```python
from build123d import *

# Parameters (mm, degrees)
F1_DEPTH = 63.4248778224
F2_R     = 5.3887909161
F3_DEPTH = 102.1241396666
F6_DEPTH = 25


with BuildPart() as f1:
    # F0 (on Top) → F1 (new body)
    with BuildSketch(Plane.XY):
        Polygon((-32.9633839428, -48.3821220696), (34.9777191877, -14.2513811588), (49.3006780744, 44.1745221615), (0, 63.3342713118), align=None)
    extrude(amount=F1_DEPTH)

    # F2 (on face) → F3 (cut)
    with BuildSketch(Plane(origin=(12.7649742408, -25.4101261271, 0), x_dir=(0.8935828585, 0.4488982902, 0), z_dir=(0.4488982902, -0.8935828585, 0))):
        with Locations((17.1215422451, 26.0495916009)):
            Circle(F2_R)
    extrude(amount=-F3_DEPTH, mode=Mode.SUBTRACT)

    # F5 (on face) → F6 (cut)
    with BuildSketch(Plane(origin=(36.2904519106, -8.8965103003, 0), x_dir=(0.2380972915, 0.9712413087, 0), z_dir=(0.9712413087, -0.2380972915, 0))):
        Polygon((48.6116707325, 8.5855266079), (41.9424623251, 42.4769595265), (-16.6801717132, 35.93596071), align=None)
    extrude(amount=-F6_DEPTH, mode=Mode.SUBTRACT)


solid = f1.part
```
Model file for the job. Use its own axes, mm. A direction names the side the tool comes from. Coordinates: 2 decimals unless noted, no trailing zeros. Order: outer loops, then holes, each group sorted by start corner. A loop starts at its lowest first (then second) coordinate and runs counter-clockwise, first axis right, second up. Notation, with made-up numbers: (80.5, 52.5) - (108.5, 52.5) arc R23 ccw to (108.5, 83.5) - close; hole circle Ø9 at (15.5, 38). An arc over 180 degrees is marked (long way). Return JSON: item names as keys, results as strings. Group by question number.
1) Flat gauge pins, fed straight in: P1, Ø3, axis at x = 6, z = 28, coming from the +Y side; P2, Ø2, axis at x = -11.5, z = 55, coming from the -Y side; P3, Ø5, axis at y = -7, z = 34.5, coming from the -X side. Where does each tip first touch, or does it go through?
2) Probe line 1 (X direction, y = 27.5, z = 21.5); line 2 (X direction, y = 8, z = 16.5); line 3 (X direction, y = 4, z = 14). List the from-to ranges inside material, lowest first. Write a range as from..to.
3) Mould opens along X. For faces 1 (the flat face through (8, 8, 0)), 2 (the flat face through (0.532, -31.556, 31.268)), 3 (the cylindrical face through (9.6, 16.42, 20.79)) say: released by +X, released by -X, zero draft, split by the parting line, or undercut.
4) Tool access for faces 4 (the flat face through (42.04, 14.55, 45.36)), 5 (the flat face through (35.11, 38.06, 25.29)): list every direction of +Z, -Z, +X, -X, +Y, -Y with a clear straight run to the whole face (end or side of a thin tool).
5) Saw through at C-C, the plane y = -38.5. Write the cut outline in (x, z).
6) Saw through at D-D, the plane z = 51. Write the cut outline in (x, y), plus the area to 3 significant figures.
7) Saw through at B-B, the plane z = 38.5. Write the cut outline in (x, y), plus the area to 3 significant figures.
8) Saw through at A-A, the plane x = 43.5. Write the cut outline in (y, z).
Values found:
{
 "1": {"P1": "stops at y = 61.59", "P2": "stops at y = -38.1", "P3": "stops at x = -21.49"},
 "2": {"line 1": "x = -10.57..2.11, 8.58..19.47", "line 2": "x = -16.33..40.43", "line 3": "x = -17.51..39.45"},
 "3": {"face 1": "zero draft", "face 2": "released by +X", "face 3": "undercut"},
 "4": {"face 4": "+Z, -Z, +X, -Y", "face 5": "none"},
 "5": {"outline": "(-30.05, 0) - (-13.29, 0) - (-13.29, 63.42) - (-30.05, 63.42) - close"},
 "6": {"outline": "(-32.96, -48.38) - (34.98, -14.25) - (49.3, 44.17) - (0, 63.33) - close", "area": "4,810 mm²"},
 "7": {"outline": "(-32.96, -48.38) - (34.98, -14.25) - (37.79, -2.78) - (13.51, 3.17) - (22.18, 38.55) - (46.46, 32.6) - (49.3, 44.17) - (0, 63.33) - close", "area": "3,900 mm²"},
 "8": {"outline": "(20.51, 0) - (46.43, 0) - (46.43, 63.42) - (20.51, 63.42) - (20.51, 41.18) - (32.52, 42.48) - (39.39, 8.59) - (20.51, 16.26) - close"}
}
